Here's how the part is built. I have some questions about the finished solid (model axes, mm). Face numbers are marked on the shaded views. A direction names the side the tool comes from. Round coordinates to 2 decimals unless told otherwise and drop trailing zeros. Write each loop counter-clockwise with the first axis right and the second up, starting at its lowest first coordinate (ties: lowest second). Pieces come first, ordered by that corner, then holes. Notation, with made-up numbers: (70.5, 14) -> (120.5, 14) arc R22 ccw to (120.5, 42) -> close; hole circle Ø5 at (42.5, 53). An arc over 180 degrees is marked (long way). Answer as CSV lines item,"result".
from build123d import *

# Parameters (mm, degrees)
BOSS_EXTRUDE1_DEPTH = 59.6
CUT_EXTRUDE1_DEPTH  = 59.6
SKETCH3_R           = 1.5000000000000004
SKETCH3_R_2         = 1.5000000000000007
SKETCH3_R_3         = 1.5000000000000009
SKETCH3_R_4         = 1.5000000000000002
CUT_EXTRUDE2_DEPTH  = 66.4
CHAMFER1_SIZE       = 1
SKETCH4_R           = 3
CUT_EXTRUDE3_DEPTH  = 66.4
FILLET1_R           = 4
CUT_EXTRUDE4_DEPTH  = 59.6
SKETCH5_R           = 10
BOSS_EXTRUDE2_DEPTH = 2
BOSS_EXTRUDE3_DEPTH = 17
CHAMFER2_SIZE       = 4
CHAMFER2_SIZE_2     = 3.038324347
CHAMFER3_SIZE       = 4
FILLET3_R           = 2
CHAMFER4_SIZE       = 14
CHAMFER5_SIZE       = 2
FILLET4_R           = 8
SKETCH11_R          = 5.000000000000001
CUT_EXTRUDE5_DEPTH  = 4


with BuildPart() as part:
    # Sketch1 → Boss-Extrude1 (new body)
    with BuildSketch(Plane(origin=(0, 0, 0), x_dir=(1, 0, 0), z_dir=(0, 1, 0))):
        with BuildLine():
            ThreePointArc((6.1e-16, 9.999999999999998), (-9.999999999999998, 1.22e-15), (-1.84e-15, -9.999999999999998))
            Line((0, -9.999999999999998), (0, 10.000000000000002))
        make_face()
        with BuildLine():
            Line((0, 10.000000000000002), (0, -9.999999999999998))
            ThreePointArc((-1.84e-15, -9.999999999999998), (7.071067811865472, -7.0710678118654755), (9.999999999999998, -2.45e-15))
            ThreePointArc((9.999999999999998, 0), (7.071067811865475, 7.071067811865474), (6.1e-16, 9.999999999999998))
        make_face()
        with BuildLine():
            ThreePointArc((9.999999999999998, -2.45e-15), (7.071067811865472, -7.0710678118654755), (-1.84e-15, -9.999999999999998))
            Line((0, -9.999999999999998), (25, -9.999999999999998))
            Line((25, -9.999999999999998), (25, 10.000000000000002))
            Line((25, 10), (0, 10.000000000000002))
            ThreePointArc((6.1e-16, 9.999999999999998), (7.071067811865475, 7.071067811865474), (9.999999999999998, 0))
        make_face()
    extrude(amount=BOSS_EXTRUDE1_DEPTH)

    # Sketch2 → Cut-Extrude1 (cut)
    with BuildSketch(Plane.XY.offset(9.999999999999998)):
        Polygon((-9.999999999999998, 4.0000000000000036), (21, 4), (21, 55.599999999999994), (-9.999999999999998, 55.599999999999994), align=None)
    extrude(amount=-CUT_EXTRUDE1_DEPTH, mode=Mode.SUBTRACT)

    # Sketch3 → Cut-Extrude2 (cut, through all)
    with BuildSketch(Plane(origin=(0, 59.6, 0), x_dir=(1, 0, 0), z_dir=(0, 1, 0))):
        with Locations(Location((-7, 0, 0), (0, 0, 270))):
            Circle(SKETCH3_R)
        with Locations(Location((2.444e-14, 7, 0), (0, 0, 270))):
            Circle(SKETCH3_R_2)
        with Locations(Location((7, -4.888e-14, 0), (0, 0, 270))):
            Circle(SKETCH3_R_3)
        with Locations(Location((-7.332e-14, -7.000000000000001, 0), (0, 0, 270))):
            Circle(SKETCH3_R_4)
    extrude(amount=-CUT_EXTRUDE2_DEPTH, mode=Mode.SUBTRACT)

    # Chamfer1
    chamfer1_edges = [part.edges().sort_by_distance(p)[0] for p in [
        (-7, 0, -1.5000000000000004),
        (-7, 59.6, -1.5000000000000004),
        (2.49e-14, 0, -8.5),
        (2.49e-14, 59.6, -8.5),
        (7.000000000000001, 0, -1.499999999999952),
        (7.000000000000001, 59.6, -1.499999999999952),
        (-7.286e-14, 0, 5.500000000000001),
        (-7.286e-14, 59.6, 5.500000000000001),
    ]]
    chamfer(chamfer1_edges, length=CHAMFER1_SIZE)

    # Sketch4 → Cut-Extrude3 (cut, through all)
    with BuildSketch(Plane(origin=(0, 59.6, 0), x_dir=(1, 0, 0), z_dir=(0, 1, 0))):
        with Locations(Location((0, 0, 0), (0, 0, 270))):
            Circle(SKETCH4_R)
    extrude(amount=-CUT_EXTRUDE3_DEPTH, mode=Mode.SUBTRACT)

    # Fillet1
    fillet1_edges = [part.edges().sort_by_distance(p)[0] for p in [
        (21, 4, -1.78e-15),
        (21, 55.599999999999994, -1.78e-15),
    ]]
    fillet(fillet1_edges, radius=FILLET1_R)

    # Sketch6 → Cut-Extrude4 (cut)
    with BuildSketch(Plane(origin=(25, 0, 0), x_dir=(0, 0, -1), z_dir=(1, 0, 0))):
        Polygon((30, 19.799999999999997), (-10, 19.799999999999983), (-9.999999999999998, 39.800000000000004), (30, 39.800000000000004), align=None)
    extrude(amount=-CUT_EXTRUDE4_DEPTH, mode=Mode.SUBTRACT)


with BuildPart() as cut_extrude4_piece_1:
    # of the separate pieces the step leaves, piece 1, a body of its own (cut_extrude4_pieces)
    add(part.part.solids().sort_by_distance((21, 39.8, -10))[0])



with BuildPart() as cut_extrude4_piece_2:
    # of the separate pieces the step leaves, piece 2, a body of its own (cut_extrude4_pieces)
    add(part.part.solids().sort_by_distance((17, 4, -10))[0])


with BuildPart() as body_3:
    # Sketch5 → Boss-Extrude2 (new, symmetric)
    with BuildSketch(Plane(origin=(1.67e-15, 29.8, 0), x_dir=(-1, 6e-17, 0), z_dir=(-6e-17, -1, 0))):
        with Locations(Location((-25, 0, 0), (0, 0, 180))):
            Circle(SKETCH5_R)
    extrude(amount=BOSS_EXTRUDE2_DEPTH, both=True)


with BuildPart() as cut_extrude4_piece_1_1:
    add(cut_extrude4_piece_1.part)

    add(cut_extrude4_piece_2.part)  # Boss-Extrude3 merges Cut-Extrude4 piece 2

    add(body_3.part)  # Boss-Extrude3 merges body 3
    # Sketch8 → Boss-Extrude3 (add, symmetric)
    with BuildSketch(Plane(origin=(1.67e-15, 29.8, 0), x_dir=(-1, 6e-17, 0), z_dir=(-6e-17, -1, 0))):
        with BuildLine():
            Line((-18.00145787776235, -7.1428571428571415), (-15.202041028867285, -9.999999999999998))
            ThreePointArc((-15.202041028867285, -9.999999999999998), (-25.14286458158996, -13.999271042140986), (-35, -9.797958971132715))
            Line((-35, -9.797958971132715), (-32.142857142857146, -6.998542122237653))
            ThreePointArc((-32.142857142857146, -6.998542122237653), (-25.10204612970712, -9.999479315814993), (-18.00145787776235, -7.1428571428571415))
        make_face()
    extrude(amount=BOSS_EXTRUDE3_DEPTH, both=True)

    # Chamfer2
    # the kernel refuses this chamfer: 4, 3.038324347 mm, written as the material it adds along each edge
    with BuildSketch(Plane(origin=(25, 39.800000000000004, 9.999999999999998), x_dir=(0, 0, -1), z_dir=(0, 1, 0))) as chamfer2_piece_1:
        with BuildLine():
            Line((CHAMFER2_SIZE, 0), (0.5968757625671461, -3.403124237432852))
            ThreePointArc((0.5968757625671461, -3.403124237432852), (0.15846004750250664, -1.7731585838259747), (0, 0))
            Line((0, 0), (CHAMFER2_SIZE, 0))
        make_face()
    extrude(amount=6.999999999999993)
    with BuildSketch(Plane(origin=(25, 12.799999999999999, 9.999999999999998), x_dir=(0.9849650815494138, 0, -0.17275354736837392), z_dir=(0, 1, 0))) as chamfer2_piece_2:
        with BuildLine():
            Line((3.4550709473675134, 2e-17), (CHAMFER2_SIZE * 0.172753547368, CHAMFER2_SIZE * 0.984965081549))
            Line((CHAMFER2_SIZE * 0.172753547368, CHAMFER2_SIZE * 0.984965081549), (0, 0))
            ThreePointArc((0, 0), (1.773873824440413, -0.15024182179198892), (3.4550709473675134, 2e-17))
        make_face()
    extrude(amount=6.999999999999984)
    with BuildSketch(Plane(origin=(21, 46.8, 9.165151389911681), x_dir=(0, 0, -1), z_dir=(-6e-17, -1, 0))) as chamfer2_piece_3:
        with BuildLine():
            Line((CHAMFER2_SIZE, 0), (1.5355475582413494, -2.464452441758805))
            ThreePointArc((1.5355475582413494, -2.464452441758805), (0.6874579868810571, -1.3036510598088036), (0, 0))
            Line((0, 0), (CHAMFER2_SIZE, 0))
        make_face()
    extrude(amount=6.999999999999993)
    with BuildSketch(Plane(origin=(21, 19.799999999999983, 9.165151389911681), x_dir=(-0.8336339896703572, 0, -0.5523172740973098), z_dir=(-6e-17, -1, 0))) as chamfer2_piece_4:
        with BuildLine():
            Line((3.4550709473675125, 1.3e-16), (CHAMFER2_SIZE_2 * 0.552317274099, CHAMFER2_SIZE_2 * 0.833633989672))
            Line((CHAMFER2_SIZE_2 * 0.552317274099, CHAMFER2_SIZE_2 * 0.833633989672), (0, 0))
            ThreePointArc((0, 0), (1.7738738244404142, -0.1502418217919865), (3.4550709473675125, 1.3e-16))
        make_face()
    extrude(amount=6.999999999999982)
    # the kernel refuses this chamfer: 4, 3.038324347 mm, written as the material it takes off along each edge
    with BuildSketch(Plane(origin=(42.3476656799026, 46.8, 16.997171657661287), x_dir=(4.2e-16, -1, -4.8e-16), z_dir=(-0.7142857142857139, 0, -0.6998542122237658))) as chamfer2_2_piece_1_section:
        Polygon((CHAMFER2_SIZE, 0), (-2.54e-15, CHAMFER2_SIZE), (0, 0), align=None)
    chamfer2_2_piece_1 = extrude(amount=24.573463903727287, mode=Mode.PRIVATE)
    chamfer2_2_piece_1 = split(chamfer2_2_piece_1, bisect_by=Plane(origin=(25, 46.8, 16.997171657661287), z_dir=(1, 0, 0)), keep=Keep.TOP, mode=Mode.PRIVATE)
    add(chamfer2_2_piece_1, mode=Mode.SUBTRACT)
    with BuildSketch(Plane(origin=(42.3476656799026, 12.799999999999999, 16.997171657661287), x_dir=(-0.6998542122237658, 0, 0.7142857142857139), z_dir=(-0.7142857142857139, 0, -0.6998542122237658))) as chamfer2_2_piece_2_section:
        Polygon((CHAMFER2_SIZE, 0), (-2.54e-15, CHAMFER2_SIZE), (0, 0), align=None)
    chamfer2_2_piece_2 = extrude(amount=24.57346390372729, mode=Mode.PRIVATE)
    chamfer2_2_piece_2 = split(chamfer2_2_piece_2, bisect_by=Plane(origin=(25, 12.799999999999999, 16.997171657661287), z_dir=(1, 0, 0)), keep=Keep.TOP, mode=Mode.PRIVATE)
    add(chamfer2_2_piece_2, mode=Mode.SUBTRACT)

    # Chamfer3
    # the kernel refuses this chamfer: 4 mm, written as the material it adds along each edge
    with BuildSketch(Plane(origin=(32.142857142857146, 31.8, 6.998542122237653), x_dir=(0.7142857142857139, 0, 0.6998542122237658), z_dir=(0, -1, 0))) as chamfer3_piece_1:
        with BuildLine():
            Line((CHAMFER3_SIZE, -9e-17), (-2.0000000000000133, -6.0000000000000115))
            ThreePointArc((-2.0000000000000133, -6.0000000000000115), (-0.5373798977418118, -3.234010018589798), (0, 0))
            Line((0, 0), (CHAMFER3_SIZE, -9e-17))
        make_face()
    extrude(amount=4)

    # Fillet3
    fillet3_edges = [cut_extrude4_piece_1_1.edges().sort_by_distance(p)[0] for p in [
        (32.142857142857146, 37.3, 6.998542122237653),
        (32.142857142857146, 22.3, 6.998542122237653),
    ]]
    fillet(fillet3_edges, radius=FILLET3_R)

    # Chamfer4
    chamfer4_edges = [cut_extrude4_piece_1_1.edges().sort_by_distance(p)[0] for p in [
        (23, 39.800000000000004, -10),
        (23, 19.79999999999999, -10),
    ]]
    chamfer(chamfer4_edges, length=CHAMFER4_SIZE)

    # Chamfer5
    chamfer5_edges = [cut_extrude4_piece_1_1.edges().sort_by_distance(p)[0] for p in [
        (23, 46.8, 9.999999999999998),
        (23, 12.8, 9.999999999999998),
    ]]
    chamfer(chamfer5_edges, length=CHAMFER5_SIZE)

    # Fillet4
    fillet4_edges = [cut_extrude4_piece_1_1.edges().sort_by_distance(p)[0] for p in [
        (25, 0, -1.78e-15),
        (25, 59.6, -1.78e-15),
    ]]
    fillet(fillet4_edges, radius=FILLET4_R)

    # Sketch11 → Cut-Extrude5 (cut)
    with BuildSketch(Plane.XZ.offset(-27.8)):
        with Locations((25, 0)):
            Circle(SKETCH11_R)
    extrude(amount=-CUT_EXTRUDE5_DEPTH, mode=Mode.SUBTRACT)


solid = cut_extrude4_piece_1_1.part
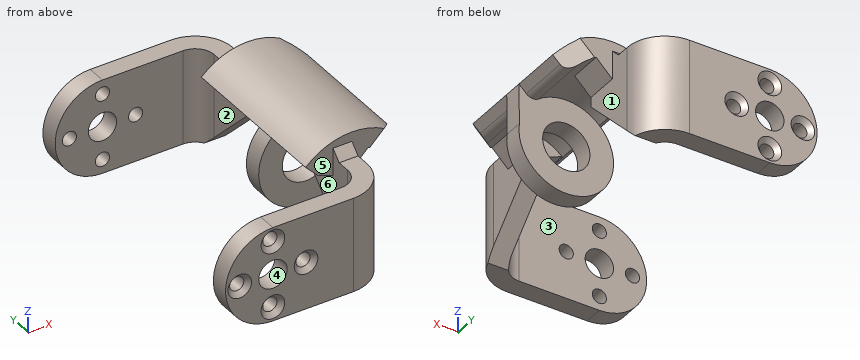
Item 1: Suppose I cut it at B-B, the plane x = 23.5. List the corners of the cut face in (y, z) for me, then the cut area to 3 significant figures.
Results found:
outline,"(3.34, -10) -> (5.8, -10) -> (19.8, 4) -> (19.8, 9.89) -> (27.8, 9.89) -> (27.8, 4.77) -> (31.8, 4.77) -> (31.8, 9.89) -> (39.8, 9.89) -> (39.8, 4) -> (53.8, -10) -> (56.26, -10) -> (56.26, 10) -> (48.8, 10) -> (46.8, 12) -> (46.8, 13.92) -> (12.8, 13.92) -> (12.8, 12) -> (10.8, 10) -> (3.34, 10) -> close; (27.8, -9.89) -> (31.8, -9.89) -> (31.8, -4.77) -> (27.8, -4.77) -> close"
area,"643 mm²"
Item 2: Suppose I cut it at C-C, the plane z = -7. State how many separate pieces and enclosed holes the cut face has, then the cut area to 3 significant figures.
Results found:
separate pieces,"5"
enclosed holes,"0"
area,"306 mm²"
Item 3: For the marked faces 1, 2 and 3, which set-ups out of +Z, -Z, +X, -X, +Y, -Y let a thin tool reach every point of the face, with its end or its side?
Results found:
face 1,"-Z, +X, +Y"
face 2,"-Z, -X"
face 3,"+Z, -Z, -X"
Item 4: If we mould it in two halves opening along X, with no side actions, what happens to the marked faces 4, 5 and 6? For each: pulls with the +X half, pulls with the -X half, needs draft (parallel to the pull), parting line crosses it, or undercut.
Results found:
face 4,"undercut"
face 5,"needs draft"
face 6,"pulls with the -X half"
Item 5: Will these pins go through, and if not, where does the flat tip stop? pin 1 (5.5 mm diameter, centred on x = 0, z = 0, fed in from +Y); pin 2 (10 mm diameter, centred on x = 18, y = 33, fed in from +Z); pin 3 (12 mm diameter, centred on x = 9, z = -0.5, fed in from +Y); pin 4 (1 mm diameter, centred on x = 30, y = 42, fed in from -Z).
Results found:
pin 1,"passes through"
pin 2,"stops at z = 13.86"
pin 3,"stops at y = 59.6"
pin 4,"stops at z = 8.35"
Item 6: Suppose I cut it at A-A, the plane y = 29. List the corners of the cut face in (x, z) for me.
Results found:
outline,"(15.2, 10) -> (18, 7.14) arc R10 ccw (long way) to (34.91, 1.31) -> (35, 9.8) arc R14 ccw to start; hole circle Ø10 at (25, 0)"
Item 7: I need wall thicknesses on L1, parallel to Y at x = 4, z = 9; L2, parallel to Y at x = 19, z = -2.25; L3, parallel to X at y = 2.7, z = -7. Which ranges of each line are inside material? Lowest first, please.
Results found:
L1,"y = 0 to 4, 55.6 to 59.6"
L2,"y = 0.25 to 4.54, 27.8 to 31.8, 55.06 to 59.35"
L3,"x = -7.14 to -1.5, 1.5 to 22.99"
Item 8: Suppose I cut it at D-D, the plane x = -7. List the corners of the cut face in (y, z) for me, then the cut area to 3 significant figures.
Results found:
outline,"(0, -7.14) -> (4, -7.14) -> (4, -1.5) -> (1, -1.5) -> (0, -2.5) -> close; (0, 2.5) -> (1, 1.5) -> (4, 1.5) -> (4, 7.14) -> (0, 7.14) -> close; (55.6, -7.14) -> (59.6, -7.14) -> (59.6, -2.5) -> (58.6, -1.5) -> (55.6, -1.5) -> close; (55.6, 1.5) -> (58.6, 1.5) -> (59.6, 2.5) -> (59.6, 7.14) -> (55.6, 7.14) -> close"
area,"88.3 mm²"
